Part model, mm, in its own coordinate system. A direction names the side the tool comes from. Round coordinates to 2 decimals unless told otherwise and drop trailing zeros. Loops run counter-clockwise (first coordinate to the right, second up) from the corner with the lowest first, then second, coordinate; pieces in that order, holes last. Notation, with made-up numbers: M 19.5,74 L 33.5,74 A23 cw 33.5,100 Z; hole C 76,84 d7. An arc over 180 degrees is marked long. Answer as CSV lines item,"result". Start each with the question number.
Item 1: Wall check: line 1 (Y direction, x = 8, z = 2); line 2 (X direction, y = 8, z = 31); line 3 (Z direction, x = 30, y = 10.25). Give the ranges that are in metal, low to high.
Item 2: Band-saw the part on B-B (z = 68). Give the cut face in (x, y).
Item 3: Which spindle directions (+Z, -Z, +X, -X, +Y, -Y) get a long thin tool onto all of the face, cutting with end or side? Do faces 4 (the cylindrical face through (17.587, 5.588, 1.972)), 5 (the flat face through (74, 5, 76.5)), 6 (the flat face through (71.5, 8, 47)). Say none if no direction does.
Item 4: Drop flat-ended pins along their axis: pin 1 Ø2.5 at (x, y) = (15.59, 5.5) entering from -Z; pin 2 Ø1.5 at (x, y) = (36, 6.5) entering from +Z; pin 3 Ø3.5 at (y, z) = (3.5, 32) entering from -X; pin 4 Ø2 at (x, y) = (73, 5.5) entering from -Z. Give the stop position or say it passes through.
Item 5: Mould opens along Z. For faces 1 (the flat face through (30, 6, 4)), 2 (the cylindrical face through (0.57, 10.4, 2.03)), 3 (the cylindrical face through (73.472, 5.588, 36.184)) say: pulls with the +Z half, pulls with the -Z half, needs draft (parallel to the pull), parting line crosses it, or undercut.
Item 6: Band-saw the part on C-C (x = 22.5). Give the cut face in (y, z).
Item 7: Band-saw the part on D-D (z = 7.5). Give the cut face in (x, y).
Item 8: Band-saw the part on A-A (x = 8). Give the cut face in (y, z).
```python
from build123d import *

# Parameters (mm, degrees)
SKETCH2_W           = 71.5
SKETCH2_H           = 11
BOSS_EXTRUDE2_DEPTH = 4
SKETCH3_R           = 2
CUT_EXTRUDE1_DEPTH  = 4
SKETCH4_W           = 4
SKETCH4_H           = 4
BOSS_EXTRUDE3_DEPTH = 11
SKETCH5_W           = 4
SKETCH5_H           = 11
BOSS_EXTRUDE4_DEPTH = 76
CUT_EXTRUDE2_DEPTH  = 4
FILLET1_R           = 10
FILLET2_R           = 10
FILLET4_R           = 2
SKETCH7_R           = 2
CUT_EXTRUDE3_DEPTH  = 4
SKETCH8_R           = 2
CUT_EXTRUDE4_DEPTH  = 4


with BuildPart() as part:
    # Sketch2 → Boss-Extrude2 (new body)
    with BuildSketch(Plane.XY):
        with Locations((35.75, 5.5)):
            Rectangle(SKETCH2_W, SKETCH2_H)
    extrude(amount=BOSS_EXTRUDE2_DEPTH)

    # Sketch3 → Cut-Extrude1 (cut)
    with BuildSketch(Plane.XY.offset(4)):
        with Locations((8, 5.5)):
            Circle(SKETCH3_R)
    extrude(amount=-CUT_EXTRUDE1_DEPTH, mode=Mode.SUBTRACT)

    # Sketch4 → Boss-Extrude3 (add)
    with BuildSketch(Plane(origin=(0, 11, 0), x_dir=(1, 0, 0), z_dir=(0, 1, 0))):
        with Locations((73.5, -2)):
            Rectangle(SKETCH4_W, SKETCH4_H)
    extrude(amount=-BOSS_EXTRUDE3_DEPTH)

    # Sketch5 → Boss-Extrude4 (add)
    with BuildSketch(Plane.XY.offset(4)):
        with Locations((73.5, 5.5)):
            Rectangle(SKETCH5_W, SKETCH5_H)
    extrude(amount=BOSS_EXTRUDE4_DEPTH)

    # Sketch6 → Cut-Extrude2 (cut)
    with BuildSketch(Plane(origin=(75.5, 0, 0), x_dir=(0, 0, -1), z_dir=(1, 0, 0))):
        with BuildLine():
            Line((-75.5, 1), (-73.5, 1))
            ThreePointArc((-73.5, 1), (-72.792893219, 1.292893219), (-72.5, 2))
            Line((-72.5, 2), (-72.5, 7.838562936))
            ThreePointArc((-72.5, 7.838562936), (-72.792893219, 8.545669717), (-73.5, 8.838562936))
            Line((-73.5, 8.838562936), (-75.5, 8.838562936))
            ThreePointArc((-75.5, 8.838562936), (-76.207106781, 8.545669717), (-76.5, 7.838562936))
            Line((-76.5, 7.838562936), (-76.5, 2))
            ThreePointArc((-76.5, 2), (-76.207106781, 1.292893219), (-75.5, 1))
        make_face()
    extrude(amount=-CUT_EXTRUDE2_DEPTH, mode=Mode.SUBTRACT)

    # Fillet1
    fillet1_edges = [part.edges().sort_by_distance(p)[0] for p in [
        (71.5, 5.5, 4),
    ]]
    fillet(fillet1_edges, radius=FILLET1_R)

    # Fillet2
    fillet2_edges = [part.edges().sort_by_distance(p)[0] for p in [
        (75.5, 5.5, 0),
    ]]
    fillet(fillet2_edges, radius=FILLET2_R)

    # Fillet4
    fillet4_edges = [part.edges().sort_by_distance(p)[0] for p in [
        (0, 11, 2),
        (0, 0, 2),
    ]]
    fillet(fillet4_edges, radius=FILLET4_R)

    # Sketch7 → Cut-Extrude3 (cut)
    with BuildSketch(Plane(origin=(0, 0, 0), x_dir=(-1, 0, 0), z_dir=(0, 0, -1))):
        with Locations((-15.588658676, 5.5)):
            Circle(SKETCH7_R)
        with Locations((-26.588658676, 5.5)):
            Circle(SKETCH7_R)
        with Locations((-37.588658676, 5.5)):
            Circle(SKETCH7_R)
        with Locations((-48.588658676, 5.5)):
            Circle(SKETCH7_R)
        with Locations((-59.588658676, 5.5)):
            Circle(SKETCH7_R)
    extrude(amount=-CUT_EXTRUDE3_DEPTH, mode=Mode.SUBTRACT)

    # Sketch8 → Cut-Extrude4 (cut)
    with BuildSketch(Plane.ZY.offset(-71.5)):
        with Locations((18.18197142, 5.5)):
            Circle(SKETCH8_R)
        with Locations((28.18197142, 5.5)):
            Circle(SKETCH8_R)
        with Locations((38.18197142, 5.5)):
            Circle(SKETCH8_R)
        with Locations((48.18197142, 5.5)):
            Circle(SKETCH8_R)
        with Locations((58.18197142, 5.5)):
            Circle(SKETCH8_R)
        with Locations((68.18197142, 5.5)):
            Circle(SKETCH8_R)
    extrude(amount=-CUT_EXTRUDE4_DEPTH, mode=Mode.SUBTRACT)


solid = part.part
```
Answer block:
1,line 1,"y = 0 to 3.5, 7.5 to 11"
1,line 2,"x = 71.5 to 75.5"
1,line 3,"z = 0 to 4"
2,outline,"M 71.5,0 L 75.5,0 L 75.5,3.51 L 71.5,3.51 Z; M 71.5,7.49 L 75.5,7.49 L 75.5,11 L 71.5,11 Z"
3,face 4,"+Z, -Z"
3,face 5,"+X, -X"
3,face 6,"+Z, -X, +Y, -Y"
4,pin 1,"passes through"
4,pin 2,"stops at z = 4"
4,pin 3,"stops at x = 71.5"
4,pin 4,"stops at z = 2.4"
5,face 1,"pulls with the +Z half"
5,face 2,"needs draft"
5,face 3,"undercut"
6,outline,"M 0,0 L 11,0 L 11,4 L 0,4 Z"
7,outline,"M 69.1,0 L 75.18,0 L 75.18,11 L 69.1,11 Z"
8,outline,"M 0,0 L 3.5,0 L 3.5,4 L 0,4 Z; M 7.5,0 L 11,0 L 11,4 L 7.5,4 Z"
